```python
from build123d import *

# Parameters (mm, degrees)
F1_DEPTH = 19.05


with BuildPart() as f1:
    # F0 (on Front) → F1 (new body)
    with BuildSketch(Plane.XZ):
        Polygon((203.910831, 97.620917), (-380.289169, 97.620917), (-380.289169, -92.879083), (-380.289169, -169.079083), (-380.289169, -359.579083), (203.910831, -359.579083), (203.910831, -169.079083), (203.910831, -92.879083), align=None)
        Polygon((-380.289169, -169.079083), (-380.289169, -92.879083), (-405.689169, -92.879083), (-405.689169, -130.979083), (-405.689169, -169.079083), align=None)
        Polygon((229.310831, -92.879083), (203.910831, -92.879083), (203.910831, -169.079083), (229.310831, -169.079083), (229.310831, -130.979083), align=None)
    extrude(amount=F1_DEPTH)


solid = f1.part
```
Can you work these out from the model? Positions are in its coordinate system, mm. A direction names the side the tool comes from. Give positions to 0.01 mm unless a question says otherwise; leave off trailing zeros. Loops run counter-clockwise (first coordinate to the right, second up) from the corner with the lowest first, then second, coordinate; pieces in that order, holes last. Notation, with made-up numbers: M 45.5,46.25 L 51.5,46.25 A20 cw 51.5,82.25 Z; hole C 83,82.25 d4. An arc over 180 degrees is marked long. One line per item, written item: value.
(1) Suppose I cut it at B-B on z = -62. List the corners of the cut face in (x, y) for me, plus the area to 3 significant figures.
Returned:
outline: M -380.29,-19.05 L 203.91,-19.05 L 203.91,0 L -380.29,0 Z
area: 11,100 mm^2
(2) I need wall thicknesses on line 1 (X direction, y = -3.5, z = -285.5). Which ranges of the line are inside material? Lowest first, please.
Returned:
line 1: -380.29 to 203.91
(3) Will these pins go through, and if not, where does the flat tip stop? pin 1 (5.5 mm diameter, centred on y = -14, z = -294.5, fed in from -X); pin 2 (9.5 mm diameter, centred on x = 212, y = -6.5, fed in from +Z); pin 3 (5.5 mm diameter, centred on x = 216.5, y = -5, fed in from -Z).
Returned:
pin 1: x = -380.29
pin 2: z = -92.88
pin 3: z = -169.08
(4) Suppose I cut it at A-A on y = -12. List the corners of the cut face in (x, z) for me.
Returned:
outline: M -405.69,-169.08 L -380.29,-169.08 L -380.29,-359.58 L 203.91,-359.58 L 203.91,-169.08 L 229.31,-169.08 L 229.31,-92.88 L 203.91,-92.88 L 203.91,97.62 L -380.29,97.62 L -380.29,-92.88 L -405.69,-92.88 Z
(5) Which directions (+Z, -Z, +X, -X, +Y, -Y) give clear straight access to the entire face, cutting with the end or side of a thin tool? Please do faces 1 (the face through (-393, -9, -169.079)), 2 (the face through (203.911, -9, -266)), 3 (the face through (203.911, -9, 1)), 4 (the face through (-380.289, -9, 4)).
Returned:
face 1: -Z, -X, +Y, -Y
face 2: -Z, +X, +Y, -Y
face 3: +Z, +X, +Y, -Y
face 4: +Z, -X, +Y, -Y
